from build123d import *

# Parameters (mm, degrees)
SKETCH2_W           = 88.9
SKETCH2_H           = 3.2004
BOSS_EXTRUDE1_DEPTH = 152.4
SKETCH3_R           = 1.1303
SKETCH3_R_2         = 6.35
CUT_EXTRUDE1_DEPTH  = 160.245032004
FILLET2_R           = 2.54


with BuildPart() as part:
    # Sketch2 → Boss-Extrude1 (new body)
    with BuildSketch(Plane.XY):
        with Locations((-1.625781684, -22.993244248)):
            Rectangle(SKETCH2_W, SKETCH2_H)
    extrude(amount=BOSS_EXTRUDE1_DEPTH)

    # Sketch3 → Cut-Extrude1 (cut, through all)
    with BuildSketch(Plane(origin=(0, -21.393044248, 0), x_dir=(-1, 0, 0), z_dir=(0, 1, 0))):
        with Locations(Location((14.833781684, 149.86, 0), (0, 0, 90))):
            Circle(SKETCH3_R)
        with Locations(Location((-11.683818316, 149.86, 0), (0, 0, 90))):
            Circle(SKETCH3_R)
        with Locations(Location((-7.619818316, 142.748, 0), (0, 0, 90))):
            Circle(SKETCH3_R_2)
        with Locations(Location((-33.478453416, 148.082, 0), (0, 0, 90))):
            Circle(SKETCH3_R)
        with Locations(Location((36.730016784, 148.082, 0), (0, 0, 90))):
            Circle(SKETCH3_R)
        with Locations(Location((-33.478453416, 4.318, 0), (0, 0, 90))):
            Circle(SKETCH3_R)
        with Locations(Location((36.730016784, 4.318, 0), (0, 0, 90))):
            Circle(SKETCH3_R)
        with Locations(Location((-18.450986138, 43.949273109, 0), (0, 0, 90))):
            Circle(SKETCH3_R)
        with Locations(Location((-18.450986138, 101.949273109, 0), (0, 0, 90))):
            Circle(SKETCH3_R)
        with Locations(Location((30.549013862, 101.949273109, 0), (0, 0, 90))):
            Circle(SKETCH3_R)
        with Locations(Location((30.549013862, 43.949273109, 0), (0, 0, 90))):
            Circle(SKETCH3_R)
        with BuildLine():
            Line((35.32929924, 12.595958552), (35.32929924, 133.302587666))
            ThreePointArc((35.32929924, 133.302587666), (38.50429924, 136.477587666), (41.67929924, 133.302587666))
            Line((41.67929924, 133.302587666), (41.67929924, 12.595958552))
            ThreePointArc((41.67929924, 12.595958552), (38.50429924, 9.420958552), (35.32929924, 12.595958552))
        make_face()
        with BuildLine():
            Line((-32.077735872, 12.595958552), (-32.077735872, 133.302587666))
            ThreePointArc((-32.077735872, 133.302587666), (-35.252735872, 136.477587666), (-38.427735872, 133.302587666))
            Line((-38.427735872, 133.302587666), (-38.427735872, 12.595958552))
            ThreePointArc((-38.427735872, 12.595958552), (-35.252735872, 9.420958552), (-32.077735872, 12.595958552))
        make_face()
    extrude(amount=-CUT_EXTRUDE1_DEPTH, mode=Mode.SUBTRACT)

    # Fillet2
    fillet2_edges = [part.edges().sort_by_distance(p)[0] for p in [
        (42.824218316, -22.993244248, 152.4),
        (-46.075781684, -22.993244248, 152.4),
        (42.824218316, -22.993244248, 0),
        (-46.075781684, -22.993244248, 0),
    ]]
    fillet(fillet2_edges, radius=FILLET2_R)


solid = part.part
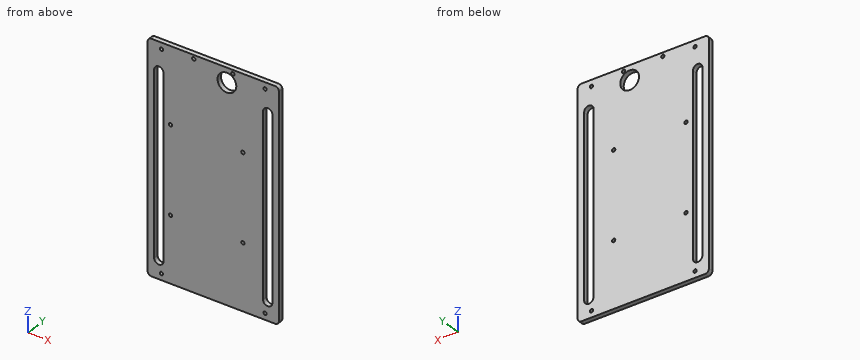
Here's how the part is built. I have some questions about the finished solid (model axes, mm). Round coordinates to 2 decimals unless told otherwise and drop trailing zeros. Write each loop counter-clockwise with the first axis right and the second up, starting at its lowest first coordinate (ties: lowest second). Pieces come first, ordered by that corner, then holes. Notation, with made-up numbers: (11.5, -25) -> (43.5, -25) arc R36 cw to (43.5, 14) -> close; hole circle Ø1 at (38, 10.5). An arc over 180 degrees is marked (long way). One line per item, written item: value.
1) Suppose I cut it at D-D on z = 138.5. List the corners of the cut face in (x, y) for me.
Filled sheet:
outline: (-46.08, -24.59) -> (2.9, -24.59) -> (2.9, -21.39) -> (-46.08, -21.39) -> close; (12.34, -24.59) -> (42.82, -24.59) -> (42.82, -21.39) -> (12.34, -21.39) -> close
2) If I drill on line 1 (X direction, y = -23, z = 130.5); line 2 (X direction, y = -23.75, z = 149.86); line 3 (Z direction, x = 12.5, y = -22.15), over which ranges is the centre line in solid material (lowest first)? Write a range as [from, to].
Filled sheet:
line 1: x = [-46.08, -41.68], [-35.33, 32.08], [38.43, 42.82]
line 2: x = [-46.08, -15.96], [-13.7, 10.55], [12.81, 42.82]
line 3: z = [0, 138.69], [146.81, 149.08], [150.64, 152.4]
3) I'm going to push a flat-ended pin straight in: pin 1 Ø1.8 at (x, z) = (-36.73, 4.32) entering from -Y. Where does the tip first touch, or does it pass through?
Filled sheet:
pin 1: passes through
4) Suppose I cut it at C-C on y = -22.35. Give the number of separate pieces and of enclosed holes in the cut face, plus the area to 3 significant figures.
Filled sheet:
separate pieces: 1
enclosed holes: 13
area: 11,800 mm2
5) Suppose I cut it at A-A on z = 51. List the corners of the cut face in (x, y) for me.
Filled sheet:
outline: (-46.08, -24.59) -> (-41.68, -24.59) -> (-41.68, -21.39) -> (-46.08, -21.39) -> close; (-35.33, -24.59) -> (32.08, -24.59) -> (32.08, -21.39) -> (-35.33, -21.39) -> close; (38.43, -24.59) -> (42.82, -24.59) -> (42.82, -21.39) -> (38.43, -21.39) -> close
6) Suppose I cut it at B-B on x = 5. List the corners of the cut face in (y, z) for me.
Filled sheet:
outline: (-24.59, 0) -> (-21.39, 0) -> (-21.39, 136.96) -> (-24.59, 136.96) -> close; (-24.59, 148.53) -> (-21.39, 148.53) -> (-21.39, 152.4) -> (-24.59, 152.4) -> close
